Can you work these out from the model? Positions are in its coordinate system, mm. Face numbers are marked on the shaded views. A direction names the side the tool comes from. Round coordinates to 2 decimals unless told otherwise and drop trailing zeros. Order: outer loops, then holes, each group sorted by start corner. A loop starts at its lowest first (then second) coordinate and runs counter-clockwise, first axis right, second up.
Q1. If we section it at A-A (x = 0): Please give me the cut outline in (y, z).
Q2. For the marked faces 4, 5 and 6, which set-ups out of +Z, -Z, +X, -X, +Y, -Y let a thin tool reach every point of the face, with its end or its side?
Q3. If we section it at D-D (x = -18): Please give me the cut outline in (y, z).
Q4. Will these pins go through, and if not, where does the flat tip stop? P1, Ø2, axis at x = 15, y = -2.5, coming from the -Z side; P2, Ø1.5, axis at y = 44.5, z = -28.5, coming from the -X side; P3, Ø3, axis at x = 17.5, z = 21.5, coming from the +Y side.
Q5. If we section it at C-C (y = 17.25): Please give me the cut outline in (x, z), plus the area to 3 significant figures.
Q6. We'd pull the mould along Z, two halves only. Please class the marked faces 1, 2 and 3: pulls with the +Z half, pulls with the -Z half, needs draft (parallel to the pull), parting line crosses it, or undercut.
Q7. If I drill on line 1 (X direction, y = -1.35, z = -23.75); line 2 (X direction, y = 17.25, z = 26.9); line 3 (Y direction, x = -23.75, z = -29), over which ranges is the centre line in solid material (lowest first)?
Q8. If we section it at B-B (y = 31): Please give me the cut outline in (x, z), plus the area to 3 significant figures.
from build123d import *

# Parameters (mm, degrees)
SKETCH_16_R                       = 2.5
SM_BASE_FLANGE_2_DEPTH            = 5
SM_EDGE_FLANGE_1_STRIP_W          = 26
SM_EDGE_FLANGE_1_STRIP_H          = 5
SM_EDGE_FLANGE_1_STRIP_CUT_DEPTH  = 27.5
SM_EDGE_FLANGE_1_RELIEF_W         = 28.5
SM_EDGE_FLANGE_1_RELIEF_H         = 2.5
SM_EDGE_FLANGE_1_RELIEF_CUT_DEPTH = 5
SM_EDGE_FLANGE_1_DEPTH            = 27.5
SM_EDGE_FLANGE_2_STRIP_W          = 26
SM_EDGE_FLANGE_2_STRIP_H          = 5
SM_EDGE_FLANGE_2_STRIP_CUT_DEPTH  = 27.5
SM_EDGE_FLANGE_2_RELIEF_W         = 28.5
SM_EDGE_FLANGE_2_RELIEF_H         = 2.5
SM_EDGE_FLANGE_2_RELIEF_CUT_DEPTH = 5
SM_EDGE_FLANGE_2_DEPTH            = 27.5
EXTRUDE_START                     = 30
SKETCH_23_W                       = 16.25
SKETCH_23_H                       = 16.25
EXTRUDE_1_DEPTH                   = 5
EXTRUDE_START_2                   = -25
SKETCH_24_W                       = 16.25
SKETCH_24_H                       = 16.25
EXTRUDE_2_DEPTH                   = 5
CUT_EXTRUDE_1_DEPTH               = 83.710337927
CUT_EXTRUDE_1_DEPTH_BACK          = 83.710337927
SKETCH_25_R                       = 2.5
CUT_EXTRUDE_2_DEPTH               = 83.710337927
CUT_EXTRUDE_2_DEPTH_BACK          = 83.710337927
SKETCH_26_R                       = 3


# Sheet-metal steps are written as plain solids
with BuildPart() as part:
    # 草图16 → 基体-法兰2 (new body)
    with BuildSketch(Plane(origin=(0, 0, 0), x_dir=(1, 0, 0), z_dir=(0, 1, 0))):
        Polygon((16.25, 30), (30, 30), (30, -30), (16.25, -30), (16.25, -25), (-16.25, -25), (-16.25, -30), (-30, -30), (-30, 30), (-16.25, 30), (-16.25, 25), (16.25, 25), align=None)
        with Locations(Location((-23.75, 23.75, 0), (0, 0, 270))):
            Circle(SKETCH_16_R, mode=Mode.SUBTRACT)
        with Locations(Location((-23.75, -23.75, 0), (0, 0, 270))):
            Circle(SKETCH_16_R, mode=Mode.SUBTRACT)
        with Locations(Location((23.75, 23.75, 0), (0, 0, 270))):
            Circle(SKETCH_16_R, mode=Mode.SUBTRACT)
        with Locations(Location((23.75, -23.75, 0), (0, 0, 270))):
            Circle(SKETCH_16_R, mode=Mode.SUBTRACT)
    extrude(amount=-SM_BASE_FLANGE_2_DEPTH)

    # 边线-法兰1 strip (across the edge) → 边线-法兰1 strip cut (cut)
    with BuildSketch(Plane(origin=(-13.75, 0, 25), x_dir=(0, 0, -1), z_dir=(1, 0, 0))):
        with Locations((-10, -2.5)):
            Rectangle(SM_EDGE_FLANGE_1_STRIP_W, SM_EDGE_FLANGE_1_STRIP_H)
    extrude(amount=SM_EDGE_FLANGE_1_STRIP_CUT_DEPTH, mode=Mode.SUBTRACT)

    # 边线-法兰1 relief (on the sheet) → 边线-法兰1 relief cut (cut)
    with BuildSketch(Plane(origin=(-13.75, 0, 22), x_dir=(0, 0, -1), z_dir=(0, 1, 0))):
        with Locations((-11.75, 1.25)):
            Rectangle(SM_EDGE_FLANGE_1_RELIEF_W, SM_EDGE_FLANGE_1_RELIEF_H)
        with Locations((-11.75, -28.75)):
            Rectangle(SM_EDGE_FLANGE_1_RELIEF_W, SM_EDGE_FLANGE_1_RELIEF_H)
    extrude(amount=-SM_EDGE_FLANGE_1_RELIEF_CUT_DEPTH, mode=Mode.SUBTRACT)

    # 边线-法兰1 section (across the edge) → 边线-法兰1 (add)
    with BuildSketch(Plane(origin=(-13.75, 0, 25), x_dir=(0, 0, -1), z_dir=(1, 0, 0))):
        with BuildLine():
            Line((-5, 3), (-5, 71))
            Line((-5, 71), (0, 71))
            Line((0, 71), (0, 3))
            ThreePointArc((0, 3), (0.878679656, 0.878679656), (3, 0))
            Line((3, 0), (3, -5))
            ThreePointArc((3, -5), (-2.656854249, -2.656854249), (-5, 3))
        make_face()
    extrude(amount=SM_EDGE_FLANGE_1_DEPTH)

    # 边线-法兰2 strip (across the edge) → 边线-法兰2 strip cut (cut)
    with BuildSketch(Plane(origin=(13.75, 0, -25), x_dir=(0, 0, 1), z_dir=(-1, 0, 0))):
        with Locations((-10, -2.5)):
            Rectangle(SM_EDGE_FLANGE_2_STRIP_W, SM_EDGE_FLANGE_2_STRIP_H)
    extrude(amount=SM_EDGE_FLANGE_2_STRIP_CUT_DEPTH, mode=Mode.SUBTRACT)

    # 边线-法兰2 relief (on the sheet) → 边线-法兰2 relief cut (cut)
    with BuildSketch(Plane(origin=(13.75, 0, -22), x_dir=(0, 0, 1), z_dir=(0, 1, 0))):
        with Locations((-11.75, 1.25)):
            Rectangle(SM_EDGE_FLANGE_2_RELIEF_W, SM_EDGE_FLANGE_2_RELIEF_H)
        with Locations((-11.75, -28.75)):
            Rectangle(SM_EDGE_FLANGE_2_RELIEF_W, SM_EDGE_FLANGE_2_RELIEF_H)
    extrude(amount=-SM_EDGE_FLANGE_2_RELIEF_CUT_DEPTH, mode=Mode.SUBTRACT)

    # 边线-法兰2 section (across the edge) → 边线-法兰2 (add)
    with BuildSketch(Plane(origin=(13.75, 0, -25), x_dir=(0, 0, 1), z_dir=(-1, 0, 0))):
        with BuildLine():
            Line((-5, 3), (-5, 71))
            Line((-5, 71), (0, 71))
            Line((0, 71), (0, 3))
            ThreePointArc((0, 3), (0.878679656, 0.878679656), (3, 0))
            Line((3, 0), (3, -5))
            ThreePointArc((3, -5), (-2.656854249, -2.656854249), (-5, 3))
        make_face()
    extrude(amount=SM_EDGE_FLANGE_2_DEPTH)

    # 草图23 → 凸台-拉伸1 (add)
    with BuildSketch(Plane.XY.offset(EXTRUDE_START)):
        with Locations((-21.875, 62.875)):
            Rectangle(SKETCH_23_W, SKETCH_23_H)
        with Locations((21.875, 62.875)):
            Rectangle(SKETCH_23_W, SKETCH_23_H)
        with Locations((21.875, 19.125)):
            Rectangle(SKETCH_23_W, SKETCH_23_H)
        with Locations((-21.875, 19.125)):
            Rectangle(SKETCH_23_W, SKETCH_23_H)
    extrude(amount=-EXTRUDE_1_DEPTH)

    # 草图24 → 凸台-拉伸2 (add)
    with BuildSketch(Plane.XY.offset(EXTRUDE_START_2)):
        with Locations((21.875, 62.875)):
            Rectangle(SKETCH_24_W, SKETCH_24_H)
        with Locations((-21.875, 62.875)):
            Rectangle(SKETCH_24_W, SKETCH_24_H)
        with Locations((-21.875, 19.125)):
            Rectangle(SKETCH_24_W, SKETCH_24_H)
        with Locations((21.875, 19.125)):
            Rectangle(SKETCH_24_W, SKETCH_24_H)
    extrude(amount=-EXTRUDE_2_DEPTH)

    # 草图25 → 切除-拉伸1 (cut, two sides: drawn at the far end of the back side and taken through both)
    with BuildSketch(Plane.XY.offset(-CUT_EXTRUDE_1_DEPTH_BACK)):
        with Locations((-23.75, 64.75)):
            Circle(SKETCH_25_R)
        with Locations((23.75, 64.75)):
            Circle(SKETCH_25_R)
        with Locations((-23.75, 17.25)):
            Circle(SKETCH_25_R)
        with Locations((23.75, 17.25)):
            Circle(SKETCH_25_R)
    extrude(amount=CUT_EXTRUDE_1_DEPTH + CUT_EXTRUDE_1_DEPTH_BACK, mode=Mode.SUBTRACT)

    # 草图26 → 切除-拉伸2 (cut, two sides: drawn at the far end of the back side and taken through both)
    with BuildSketch(Plane.XY.offset(-CUT_EXTRUDE_2_DEPTH_BACK)):
        with Locations((0, 51)):
            Circle(SKETCH_26_R)
        with Locations((0, 31)):
            Circle(SKETCH_26_R)
    extrude(amount=CUT_EXTRUDE_2_DEPTH + CUT_EXTRUDE_2_DEPTH_BACK, mode=Mode.SUBTRACT)


solid = part.part
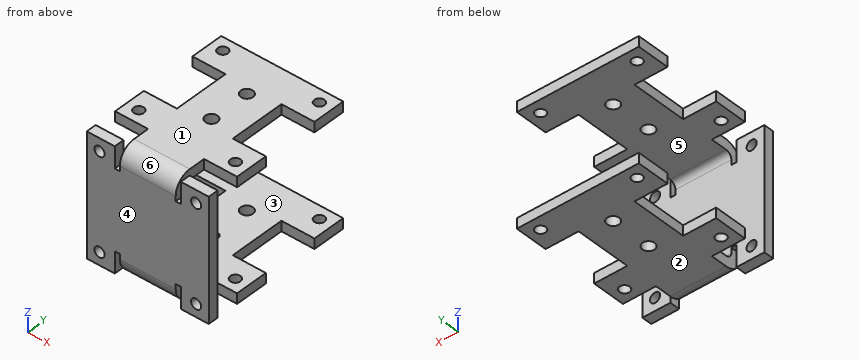
Solution:
1. outline: (-5, -22) arc R8 ccw to (3, -30) - (28, -30) - (28, -25) - (3, -25) arc R3 cw to (0, -22) - (0, 22) arc R3 cw to (3, 25) - (28, 25) - (28, 30) - (3, 30) arc R8 ccw to (-5, 22) - close; (34, -30) - (48, -30) - (48, -25) - (34, -25) - close; (34, 25) - (48, 25) - (48, 30) - (34, 30) - close; (54, -30) - (71, -30) - (71, -25) - (54, -25) - close; (54, 25) - (71, 25) - (71, 30) - (54, 30) - close
2. face 4: +Z, -Z, +X, -X, -Y
2. face 5: +X, -X, +Y
2. face 6: +Z, -Y
3. outline: (-5, -30) - (0, -30) - (0, 30) - (-5, 30) - close; (11, -30) - (27.25, -30) - (27.25, -25) - (11, -25) - close; (11, 25) - (27.25, 25) - (27.25, 30) - (11, 30) - close; (54.75, -30) - (71, -30) - (71, -25) - (54.75, -25) - close; (54.75, 25) - (71, 25) - (71, 30) - (54.75, 30) - close
4. P1: stops at z = -19.5
4. P2: stops at x = -13.75
4. P3: stops at y = 0
5. outline: (-30, -30) - (-26.25, -30) - (-26.25, -25) - (-30, -25) - close; (-30, 25) - (-26.25, 25) - (-26.25, 30) - (-30, 30) - close; (-21.25, -30) - (21.25, -30) - (21.25, -25) - (-21.25, -25) - close; (-21.25, 25) - (21.25, 25) - (21.25, 30) - (-21.25, 30) - close; (26.25, -30) - (30, -30) - (30, -25) - (26.25, -25) - close; (26.25, 25) - (30, 25) - (30, 30) - (26.25, 30) - close
5. area: 500 mm2
6. face 1: pulls with the +Z half
6. face 2: pulls with the -Z half
6. face 3: undercut
7. line 1: x = -30 to -26.25, -21.25 to -16.25, -13.75 to 13.75, 16.25 to 21.25, 26.25 to 30
7. line 2: x = -30 to -26.25, -21.25 to 21.25, 26.25 to 30
7. line 3: y = -5 to 0, 11 to 14.75, 19.75 to 27.25, 54.75 to 62.25, 67.25 to 71
8. outline: (-13.75, -30) - (-3, -30) - (-3, -25) - (-13.75, -25) - close; (-13.75, 25) - (-3, 25) - (-3, 30) - (-13.75, 30) - close; (3, -30) - (13.75, -30) - (13.75, -25) - (3, -25) - close; (3, 25) - (13.75, 25) - (13.75, 30) - (3, 30) - close
8. area: 215 mm2
